```python
from build123d import *

# Parameters (mm, degrees)
F1_DEPTH = 130
F2_SIZE  = 25
F4_D     = 24
F6_D     = 14
F7_R     = 10
F8_R     = 5


with BuildPart() as f1:
    # F0 (on Front) → F1 (new body)
    with BuildSketch(Plane.XZ):
        with BuildLine():
            Line((15, 70), (0, 70))
            Line((0, 70), (0, 25))
            ThreePointArc((0, 25), (-7.3223304703, 7.3223304703), (-25, 0))
            Line((-25, 0), (-80, 0))
            Line((-80, 0), (-80, -15))
            Line((-80, -15), (-25, -15))
            ThreePointArc((-25, -15), (3.2842712475, -3.2842712475), (15, 25))
            Line((15, 25), (15, 70))
        make_face()
    extrude(amount=F1_DEPTH)

    # F2
    f2_edges = [f1.edges().sort_by_distance(p)[0] for p in [
        (-80, -130, -7.5),
        (-80, 0, -7.5),
    ]]
    chamfer(f2_edges, length=F2_SIZE)

    # F4 (through all)
    with Locations(Plane.XY):
        with Locations((-52, -65)):
            Hole(F4_D / 2)

    # F6 (through all)
    with Locations(Plane.YZ.offset(15)):
        with Locations((-105, 45), (-25, 45)):
            Hole(F6_D / 2)

    # F7
    f7_edges = [f1.edges().sort_by_distance(p)[0] for p in [
        (-55, 0, -7.5),
        (-80, -25, -7.5),
        (-80, -105, -7.5),
        (-55, -130, -7.5),
    ]]
    fillet(f7_edges, radius=F7_R)

    # F8
    f8_edges = [f1.edges().sort_by_distance(p)[0] for p in [
        (7.5, -130, 70),
        (7.5, 0, 70),
    ]]
    fillet(f8_edges, radius=F8_R)


solid = f1.part
```
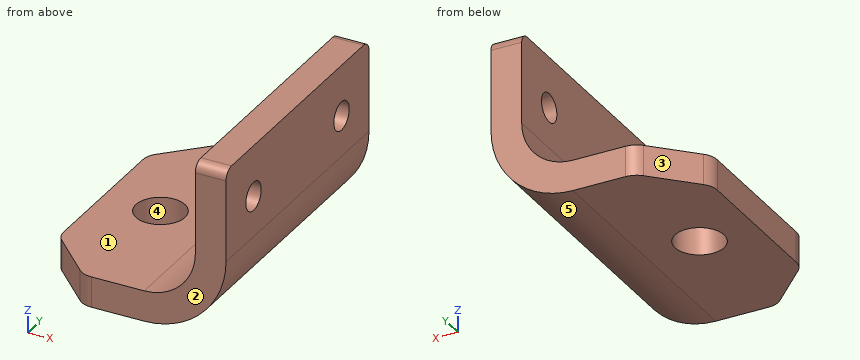
Geometry check sheet. Reference: the model listing, model coordinates, mm. Face numbers are marked on the shaded views. A direction names the side the tool comes from. Round coordinates to 2 decimals unless told otherwise and drop trailing zeros. Loops run counter-clockwise (first coordinate to the right, second up) from the corner with the lowest first, then second, coordinate; pieces in that order, holes last. Notation, with made-up numbers: (46, 7) - (88, 7) arc R13 ccw to (88, 26) - close; hole circle Ø11 at (-20, 57.5). An arc over 180 degrees is marked (long way). Write item = value, one per line. Start each with the question number.
1. Section check B-B on y = -65. Enter the section's corners in (x, z).
2. Section check C-C on y = -41. Enter the section's corners in (x, z), then the cut area to 3 significant figures.
3. Mould release check, pull along Y, two halves, no side actions. Record for the marked faces 3, 4 and 5: released by +Y, released by -Y, zero draft, split by the parting line, or undercut.
4. Depth check by flat-ended pin: pin 1 (16 mm diameter, centred on y = -25, z = 45, fed in from -X); pin 2 (16.5 mm diameter, centred on x = -55, y = -88, fed in from +Z); pin 3 (5 mm diameter, centred on y = -66.5, z = 11.5, fed in from -X). Enter the tip coordinate at first touch or a pass-through.
5. Thickness scan on line 1 (Z direction, x = -32, y = -86); line 2 (X direction, y = -17, z = 56); line 3 (Y direction, x = -52, z = -5). Record the ranges inside material, lowest first.
6. Section check A-A on z = 45. Enter the section's corners in (x, y).
7. Section check D-D on x = -60. Enter the section's corners in (y, z), then the cut area to 3 significant figures.
8. Set-up check for the marked faces 1 and 2: record each of +Z, -Z, +X, -X, +Y, -Y from which the full face is reachable in a straight line by a thin tool's end or side.
Working result:
q1.outline = (-80, -15) - (-64, -15) - (-64, 0) - (-80, 0) - close; (-40, -15) - (-25, -15) arc R40 ccw to (15, 25) - (15, 70) - (0, 70) - (0, 25) arc R25 cw to (-25, 0) - (-40, 0) - close
q2.outline = (-80, -15) - (-25, -15) arc R40 ccw to (15, 25) - (15, 70) - (0, 70) - (0, 25) arc R25 cw to (-25, 0) - (-80, 0) - close
q2.area = 2,270 mm^2
q3.face_3 = released by +Y
q3.face_4 = undercut
q3.face_5 = zero draft
q4.pin_1 = 0
q4.pin_2 = 0
q4.pin_3 = -5.79
q5.line_1 = -15 to 0
q5.line_2 = 0 to 15
q5.line_3 = -129.93 to -77, -53 to -0.07
q6.outline = (0, -130) - (15, -130) - (15, -112) - (0, -112) - close; (0, -98) - (15, -98) - (15, -32) - (0, -32) - close; (0, -18) - (15, -18) - (15, 0) - (0, 0) - close
q7.outline = (-125, -15) - (-73.94, -15) - (-73.94, 0) - (-125, 0) - close; (-56.06, -15) - (-5, -15) - (-5, 0) - (-56.06, 0) - close
q7.area = 1,530 mm^2
q8.face_1 = +Z, -X, +Y, -Y
q8.face_2 = +Z, -Z, +X, -X, -Y
